Build history of the part. All positions in model axes, mm. Face numbers are marked on the shaded views. A direction names the side the tool comes from. Give positions to 0.01 mm unless a question says otherwise; leave off trailing zeros. Order: outer loops, then holes, each group sorted by start corner. A loop starts at its lowest first (then second) coordinate and runs counter-clockwise, first axis right, second up. Notation, with made-up numbers: (-1.5, 18.5) - (28.5, 18.5) arc R28 cw to (28.5, 50.5) - close; hole circle Ø9 at (8.25, 69.5). An arc over 180 degrees is marked (long way). One line per item, written item: value.
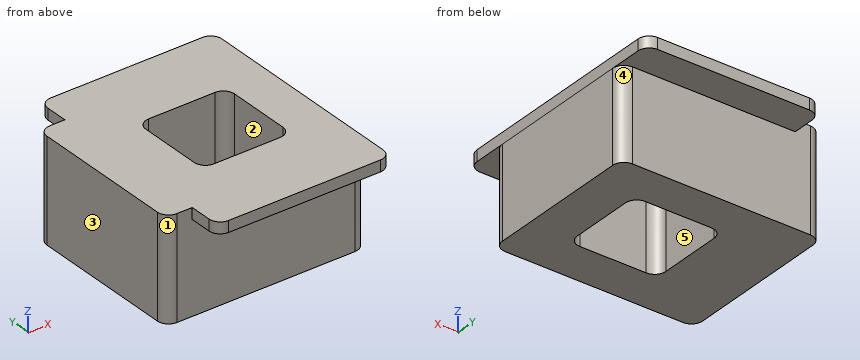
Autodesk Inventor part; units mm, degrees
ref_plane "YZ Plane" through (0, 0, 0) normal (1, 0, 0) x (0, 1, 0)
ref_plane "XZ Plane" through (0, 0, 0) normal (0, 1, 0) x (-1, 0, 0)
ref_plane "XY Plane" through (0, 0, 0) normal (0, 0, 1) x (1, 0, 0)
ref_plane "Work Plane1" through (0, 0, 0) normal (0, 0, 1) x (1, 0, 0)
sketch "Sketch1" plane through (0, 0, 0) normal (0, 0, 1) x (1, 0, 0)
  line L0 (-199.8571, 167.3322) -> (-0.3512, 153.2823)
  line L1 (-199.8571, 167.3322) -> (-212.6962, -14.9789)
  line L2 (-204.4935, -14.4012) -> (-212.6962, -14.9789)
  arc A0 (-204.4935, -14.4012) -> (-199.8571, -9.0623) centre (-204.8448, -9.4136) ccw
  line L3 (-0.3512, 4.9876) -> (-199.8571, -9.0623)
  line L4 (-0.3512, 4.9876) -> (-5.573, 79.1349)
  line L5 (-0.3512, 153.2823) -> (-5.573, 79.1349)
  line L6 (-21.5243, 154.0691) -> (-180.8464, 154.0691)
  line L7 (-190.8464, 144.0691) -> (-190.8464, 14.2008)
  line L8 (-180.8464, 4.2008) -> (-21.5243, 4.2008)
  line L9 (-11.5243, 14.2008) -> (-11.5243, 144.0691)
  circle A1 centre (-89.3933, 80.4886) radius 30.8095
  line L10 (-59.7137, 118.9158) -> (-119.0729, 118.9158)
  line L11 (-129.0729, 108.9158) -> (-129.0729, 52.0613)
  line L12 (-119.0729, 42.0613) -> (-59.7137, 42.0613)
  line L13 (-49.7137, 52.0613) -> (-49.7137, 108.9158)
  line L14 (-49.7137, 118.9158) -> (-129.0729, 42.0613) construction
  line L15 (-129.0729, 118.9158) -> (-49.7137, 42.0613) construction
  arc A2 (-49.7137, 108.9158) -> (-59.7137, 118.9158) centre (-59.7137, 108.9158) ccw
  arc A3 (-59.7137, 42.0613) -> (-49.7137, 52.0613) centre (-59.7137, 52.0613) ccw
  arc A4 (-129.0729, 52.0613) -> (-119.0729, 42.0613) centre (-119.0729, 52.0613) ccw
  arc A5 (-119.0729, 118.9158) -> (-129.0729, 108.9158) centre (-119.0729, 108.9158) ccw
  arc A6 (-11.5243, 144.0691) -> (-21.5243, 154.0691) centre (-21.5243, 144.0691) ccw
  arc A7 (-21.5243, 4.2008) -> (-11.5243, 14.2008) centre (-21.5243, 14.2008) ccw
  arc A8 (-190.8464, 14.2008) -> (-180.8464, 4.2008) centre (-180.8464, 14.2008) ccw
  arc A9 (-180.8464, 154.0691) -> (-190.8464, 144.0691) centre (-180.8464, 144.0691) ccw
  point P0 (0, 0)
  point P1 (-11.5243, 154.0691)
  point P2 (-11.5243, 4.2008)
  dimension "d0" = 10
extrude "Extrusion1" add sketch "Sketch1" along normal up to surface (81.1444 mm away) contours A6 L9 A7 L8 A8 L7 A9 L6
sketch "Sketch2" plane through (-180.8464, 154.0691, 81.1444) normal (0, 0, 1) x (1, 0, 0)
  arc A0 (121.1327, -112.0078) -> (131.1327, -102.0078) centre (121.1327, -102.0078) ccw
  line L0 (61.7735, -112.0078) -> (121.1327, -112.0078)
  arc A1 (51.7735, -102.0078) -> (61.7735, -112.0078) centre (61.7735, -102.0078) ccw
  line L1 (51.7735, -45.1533) -> (51.7735, -102.0078)
  arc A2 (61.7735, -35.1533) -> (51.7735, -45.1533) centre (61.7735, -45.1533) ccw
  line L2 (121.1327, -35.1533) -> (61.7735, -35.1533)
  arc A3 (131.1327, -45.1533) -> (121.1327, -35.1533) centre (121.1327, -45.1533) ccw
  line L3 (131.1327, -102.0078) -> (131.1327, -45.1533)
  arc A4 (159.322, -149.8683) -> (169.322, -139.8683) centre (159.322, -139.8683) ccw
  line L4 (169.322, -10) -> (169.322, -139.8683)
  arc A5 (169.322, -10) -> (159.322, 0) centre (159.322, -10) ccw
  line L5 (0, 0) -> (159.322, 0)
  arc A6 (0, 0) -> (-10, -10) centre (0, -10) ccw
  line L6 (-10, -139.8683) -> (-10, -10)
  arc A7 (-10, -139.8683) -> (0, -149.8683) centre (0, -139.8683) ccw
  line L7 (159.322, -149.8683) -> (0, -149.8683)
  line L8 (23.5841, -179.6476) -> (159.322, -179.6476)
  line L9 (169.322, -169.6476) -> (169.322, 19.7793)
  line L10 (159.322, 29.7793) -> (23.5841, 29.7793)
  line L11 (13.5841, 19.7793) -> (13.5841, -169.6476)
  line L12 (13.5841, -179.6476) -> (169.322, 29.7793) construction
  line L13 (169.322, -179.6476) -> (13.5841, 29.7793) construction
  arc A8 (169.322, 19.7793) -> (159.322, 29.7793) centre (159.322, 19.7793) ccw
  arc A9 (23.5841, 29.7793) -> (13.5841, 19.7793) centre (23.5841, 19.7793) ccw
  arc A10 (13.5841, -169.6476) -> (23.5841, -179.6476) centre (23.5841, -169.6476) ccw
  arc A11 (159.322, -179.6476) -> (169.322, -169.6476) centre (159.322, -169.6476) ccw
  point P0 (180.8464, -154.0691)
  point P1 (91.4531, -74.9342)
  dimension "d3" = 10
extrude "Extrusion2" add sketch "Sketch2" along normal blind 10
properties part number "00_Axiovert_focusblock"
(1) Pull direction Y, two halves, no side cores. Call the marked faces 3, 4 and 5: +Y half, -Y half, draft (parallel to the pull), parting line (faces both ways), or undercut.
Completed:
face 3: draft
face 4: +Y half
face 5: undercut
(2) Slice it at B-B, the plane z = 53. Give the cut face in (x, y), and give its area (3 significant figures).
Completed:
outline: (-190.85, 14.2) arc R10 ccw to (-180.85, 4.2) - (-21.52, 4.2) arc R10 ccw to (-11.52, 14.2) - (-11.52, 144.07) arc R10 ccw to (-21.52, 154.07) - (-180.85, 154.07) arc R10 ccw to (-190.85, 144.07) - close; hole (-129.07, 52.06) arc R10 ccw to (-119.07, 42.06) - (-59.71, 42.06) arc R10 ccw to (-49.71, 52.06) - (-49.71, 108.92) arc R10 ccw to (-59.71, 118.92) - (-119.07, 118.92) arc R10 ccw to (-129.07, 108.92) - close
area: 20,800 mm²
(3) Slice it at C-C, the plane y = 104. Give the cut face in (x, z).
Completed:
outline: (-190.85, 0) - (-129.07, 0) - (-129.07, 91.14) - (-190.85, 91.14) - close; (-49.71, 0) - (-11.52, 0) - (-11.52, 91.14) - (-49.71, 91.14) - close
(4) Slice it at A-A, the plane x = -74. Give the cut face in (y, z), and give its area (3 significant figures).
Completed:
outline: (-25.58, 81.14) - (4.2, 81.14) - (4.2, 0) - (42.06, 0) - (42.06, 91.14) - (-25.58, 91.14) - close; (118.92, 0) - (154.07, 0) - (154.07, 81.14) - (183.85, 81.14) - (183.85, 91.14) - (118.92, 91.14) - close
area: 7,250 mm²
(5) Drill centre lines: line 1 (X direction, y = 95, z = 78.5); line 2 (Y direction, x = -80.5, z = 9); line 3 (Y direction, x = -31, z = 49). Where is each one in solid material? Low to high.
Completed:
line 1: -190.85 to -129.07, -49.71 to -11.52
line 2: 4.2 to 42.06, 118.92 to 154.07
line 3: 4.2 to 154.07
(6) Slice it at D-D, the plane x = -26. Give the cut face in (y, z).
Completed:
outline: (-25.58, 81.14) - (4.2, 81.14) - (4.2, 0) - (154.07, 0) - (154.07, 81.14) - (183.85, 81.14) - (183.85, 91.14) - (-25.58, 91.14) - close
(7) Pin check, flat tips, straight feed: P1, Ø8, axis at x = -51.5, z = 14.5, coming from the -Y side; P2, Ø10, axis at x = -94, z = 25.5, coming from the +Y side; P3, Ø3, axis at y = -5, z = 86, coming from the -X side. Stop position of each tip, or through.
Completed:
P1: y = 4.2
P2: y = 154.07
P3: x = -167.26
(8) 3-axis set-ups, long thin cutter, end or side, ignore diameter. For the marked faces 1 and 2: which of +Z, -Z, +X, -X, +Y, -Y reach the whole face in a straight line?
Completed:
face 1: +Z, -Z, -X, -Y
face 2: +Z, -Z
